Read the model definition and answer for the solid it produces. Units are mm, in the model's axes. A direction names the side the tool comes from. Round coordinates to 2 decimals unless told otherwise and drop trailing zeros. Write each loop counter-clockwise with the first axis right and the second up, starting at its lowest first coordinate (ties: lowest second). Pieces come first, ordered by that corner, then holes. Notation, with made-up numbers: (57.25, -16.75) - (89.25, -16.75) arc R22 cw to (89.25, -2.75) - close; hole circle Ø8 at (20, 70.5). An arc over 180 degrees is marked (long way). One line per item, written item: value. Start each with the question number.
(1) The mould has two halves that part along X. Classify faces 1 (the face through (-56.996, 0.44, 34.86)), 2 (the face through (-70, 0, 12)), 3 (the face through (0, 0, 45)), 4 (the face through (-2.17, -9.76, 34.86)): +X half, -X half, draft (parallel to the pull), parting line (faces both ways), or undercut.
(2) A cutting plane is placed at C-C, the plane x = 0. Determine the outline of the cut face in (y, z).
(3) Flat-ended cylindrical pins translate along their axes: pin 1 Ø10 at (x, y) = (-38.5, 16.5) entering from +Z; pin 2 Ø4 at (x, z) = (-44.5, 35) entering from -Y; pin 3 Ø6 at (x, z) = (26, 34) entering from +Y. Find the tip coordinate at first contact, or state that the pin passes through.
(4) For faces 5 (the face through (-1, 14, 25)), 6 (the face through (-1, 30, 12)), determine the directions among +Z, -Z, +X, -X, +Y, -Y from which every point of the face is accessible in a straight line to the end or side of a thin tool.
(5) A cutting plane is placed at A-A, the plane y = 0. Determine the outline of the cut face in (x, z).
(6) Find the intervals of material crossed by L1, parallel to Z at x = -50, y = -19; L2, parallel to X at y = 4.5, z = 41.5; L3, parallel to X at y = 1.5, z = 40, in increasing order.
(7) A cutting plane is placed at B-B, the plane z = 27. Determine the outline of the cut face in (x, y).
(8) A cutting plane is placed at D-D, the plane x = 35. Determine the outline of the cut face in (y, z).
from build123d import *

# Parameters (mm, degrees)
F0_W     = 140
F0_H     = 60
F1_DEPTH = 25
F2_R     = 10
F5_DEPTH = 20
F3_R     = 10
F6_DEPTH = 20
F4_R     = 10
F7_DEPTH = 20


with BuildPart() as f1:
    # F0 (on Top) → F1 (new body)
    with BuildSketch(Plane.XY):
        Rectangle(F0_W, F0_H)
    extrude(amount=F1_DEPTH)

    # F2 (on face) → F5 (join)
    with BuildSketch(Plane.XY.offset(25)):
        with Locations((-47.00553, 0)):
            Circle(F2_R)
    extrude(amount=F5_DEPTH)

    # F3 (on face) → F6 (join)
    with BuildSketch(Plane.XY.offset(25)):
        Circle(F3_R)
    extrude(amount=F6_DEPTH)

    # F4 (on face) → F7 (join)
    with BuildSketch(Plane.XY.offset(25)):
        with Locations((30.194177, 0)):
            Circle(F4_R)
    extrude(amount=F7_DEPTH)


solid = f1.part
Here are the results:
1. face 1: undercut
1. face 2: -X half
1. face 3: draft
1. face 4: undercut
2. outline: (-30, 0) - (30, 0) - (30, 25) - (10, 25) - (10, 45) - (-10, 45) - (-10, 25) - (-30, 25) - close
3. pin 1: z = 25
3. pin 2: y = -9.99
3. pin 3: y = 9.93
4. face 5: +Z
4. face 6: +Z, -Z, +X, -X, +Y
5. outline: (-70, 0) - (70, 0) - (70, 25) - (40.19, 25) - (40.19, 45) - (20.19, 45) - (20.19, 25) - (10, 25) - (10, 45) - (-10, 45) - (-10, 25) - (-37.01, 25) - (-37.01, 45) - (-57.01, 45) - (-57.01, 25) - (-70, 25) - close
6. L1: 0 to 25
6. L2: -55.94 to -38.08, -8.93 to 8.93, 21.26 to 39.12
6. L3: -56.89 to -37.12, -9.89 to 9.89, 20.31 to 40.08
7. outline: circle Ø20 at (-47.01, 0); circle Ø20 at (0, 0); circle Ø20 at (30.19, 0)
8. outline: (-30, 0) - (30, 0) - (30, 25) - (8.77, 25) - (8.77, 45) - (-8.77, 45) - (-8.77, 25) - (-30, 25) - close
